```python
from build123d import *

# Parameters (mm, degrees)
F1_W     = 138.843298
F1_H     = 95.578349
F2_DEPTH = 15
F3_R     = 12.9
F3_W     = 65.3
F3_H     = 16.3
F3_R_2   = 7.35
F3_R_3   = 16.125
F4_DEPTH = 10
F5_R     = 5


with BuildPart() as f2:
    # F1 (on Top) → F2 (new body)
    with BuildSketch(Plane.XY):
        with Locations((-4.834347, 3.827586)):
            Rectangle(F1_W, F1_H)
    extrude(amount=F2_DEPTH)

    # F3 (on face) → F4 (cut)
    with BuildSketch(Plane.XY.offset(15)):
        with Locations((10.097019, 0)):
            Circle(F3_R)
        with Locations((-32.741672, 27.800055)):
            Rectangle(F3_W, F3_H)
        with Locations((-19.902981, 0)):
            Circle(F3_R)
        with Locations((40.097019, 0)):
            Circle(F3_R)
        with Locations((-49.902981, 0)):
            Circle(F3_R)
        with Locations((48.471941, 28.214054)):
            Circle(F3_R_2)
        with Locations((-5.631315, -27.163423)):
            Circle(F3_R)
        with Locations((-35.1047, -26.528409)):
            Circle(F3_R)
        with Locations((22.900803, 30.567518)):
            Circle(F3_R_3)
        with Locations((24.226132, -27.163423)):
            Circle(F3_R)
    extrude(amount=-F4_DEPTH, mode=Mode.SUBTRACT)

    # F5
    f5_edges = [f2.edges().sort_by_distance(p)[0] for p in [
        (64.587302, -43.961589, 7.5),
        (-74.255996, -43.961589, 7.5),
        (64.587302, 51.61676, 7.5),
        (-74.255996, 51.61676, 7.5),
    ]]
    fillet(f5_edges, radius=F5_R)


solid = f2.part
```
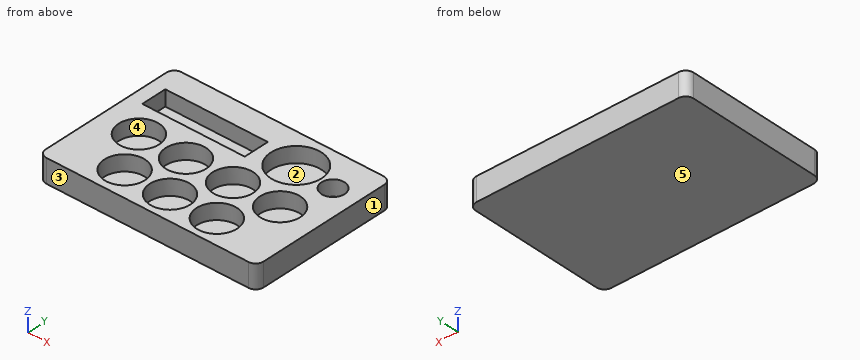
Geometry check sheet. Reference: the model listing, model coordinates, mm. Face numbers are marked on the shaded views. A direction names the side the tool comes from. Coordinates: 2 decimals unless noted, no trailing zeros. Order: outer loops, then holes, each group sorted by start corner. A loop starts at its lowest first (then second) coordinate and runs counter-clockwise, first axis right, second up. Notation, with made-up numbers: (57, 25) - (93, 25) arc R24 cw to (93, 51) - close; hole circle Ø1 at (4, 67). An arc over 180 degrees is marked (long way). Answer as a JSON object with one key per item and string values. Group by question number.
Item 1: Sectioned sample at C-C, the plane y = 11. Record the cut outline in (x, z), and give its area (3 significant figures).
Item 2: Tool access check on the marked faces 4 and 5. Record the directions out of +Z, -Z, +X, -X, +Y, -Y that give a thin tool (end or side, any length) a straight path to the whole face; none if there is none.
Item 3: Scan lines: probe 1 along Y at (x, z) = (-6, 7.25); probe 2 along Y at (x, z) = (-27, 8.5); probe 3 along X at (y, z) = (-26, 11.25). Record each from-to range of solid material in increasing order.
Item 4: Sectioned sample at A-A, the plane y = 0. Record the cut outline in (x, z).
Item 5: Sectioned sample at D-D, the plane x = -46.5. Record the cut outline in (y, z).
Item 6: Draft check along X on the marked faces 1, 2 and 3. Enter one of: +X half, -X half, draft (parallel to the pull), parting line (faces both ways), or undercut.
Item 7: Depth check by flat-ended pin: pin 1 Ø12 at (x, y) = (-2, -26.5) entering from +Z. Enter the tip coordinate at first touch or a pass-through.
Item 8: Sectioned sample at B-B, the plane x = 47. Record the cut outline in (y, z), and give its area (3 significant figures).
Resolved:
{
 "1": {"outline": "(-74.26, 0) - (64.59, 0) - (64.59, 15) - (46.84, 15) - (46.84, 5) - (33.36, 5) - (33.36, 15) - (16.84, 15) - (16.84, 5) - (3.36, 5) - (3.36, 15) - (-13.16, 15) - (-13.16, 5) - (-26.64, 5) - (-26.64, 15) - (-43.16, 15) - (-43.16, 5) - (-56.64, 5) - (-56.64, 15) - (-74.26, 15) - close", "area": "1,540 mm^2"},
 "2": {"face 4": "+Z", "face 5": "-Z, +X, -X, +Y, -Y"},
 "3": {"probe 1": "-43.96 to -40.06, -14.27 to 19.65, 35.95 to 51.62", "probe 2": "-43.96 to -36.56, -16.49 to -10.77, 10.77 to 19.65, 35.95 to 51.62", "probe 3": "-74.26 to -47.99, -22.22 to -18.48, 7.22 to 11.38, 37.07 to 64.59"},
 "4": {"outline": "(-74.26, 0) - (64.59, 0) - (64.59, 15) - (53, 15) - (53, 5) - (27.2, 5) - (27.2, 15) - (23, 15) - (23, 5) - (-2.8, 5) - (-2.8, 15) - (-7, 15) - (-7, 5) - (-32.8, 5) - (-32.8, 15) - (-37, 15) - (-37, 5) - (-62.8, 5) - (-62.8, 15) - (-74.26, 15) - close"},
 "5": {"outline": "(-43.96, 0) - (51.62, 0) - (51.62, 15) - (35.95, 15) - (35.95, 5) - (19.65, 5) - (19.65, 15) - (12.44, 15) - (12.44, 5) - (-12.44, 5) - (-12.44, 15) - (-20.48, 15) - (-20.48, 5) - (-32.57, 5) - (-32.57, 15) - (-43.96, 15) - close"},
 "6": {"face 1": "+X half", "face 2": "undercut", "face 3": "draft"},
 "7": {"pin 1": "z = 5"},
 "8": {"outline": "(-43.96, 0) - (51.62, 0) - (51.62, 15) - (35.42, 15) - (35.42, 5) - (21.01, 5) - (21.01, 15) - (10.9, 15) - (10.9, 5) - (-10.9, 5) - (-10.9, 15) - (-43.96, 15) - close", "area": "1,070 mm^2"}
}
